Design review of the part shown in the three views and the two pictorial views. Dimensions are in mm from the part's minimum x, y and z. A direction names the side the tool comes from. Coordinates: 2 decimals unless noted, no trailing zeros. Write each loop counter-clockwise with the first axis right and the second up, starting at its lowest first coordinate (ties: lowest second). Pieces come first, ordered by that corner, then holes. Notation, with made-up numbers: (21, 16.25) -> (57, 16.25) arc R13 ccw to (57, 39.25) -> close; hole circle Ø2 at (77.5, -8). An arc over 180 degrees is marked (long way). Answer in a Markdown table with one row per item. Add a question column.
Item 1: Take a section at C-C, the plane z = 9.75. Write out the cut boundary in (x, y).
Item 2: For the marked faces 5 and 6, list the 3-axis set-ups (+Z, -Z, +X, -X, +Y, -Y) from which the entire face can be reached by the end or side of a thin tool; tool diameter is ignored.
Item 3: Draft analysis for pull direction X (two halves, no side actions). For the marked faces 1, 2, 3 and 4, state which applies: released by +X, released by -X, zero draft, split by the parting line, or undercut.
Item 4: To check wall thickness, follow line 1 (X direction, y = 83, z = 13); line 2 (Y direction, x = 57.15, z = 1.55). State the ranges of each line that lie inside material, in increasing order.
Item 5: Take a section at A-A, the plane y = 57.15. Write out the cut boundary in (x, z).
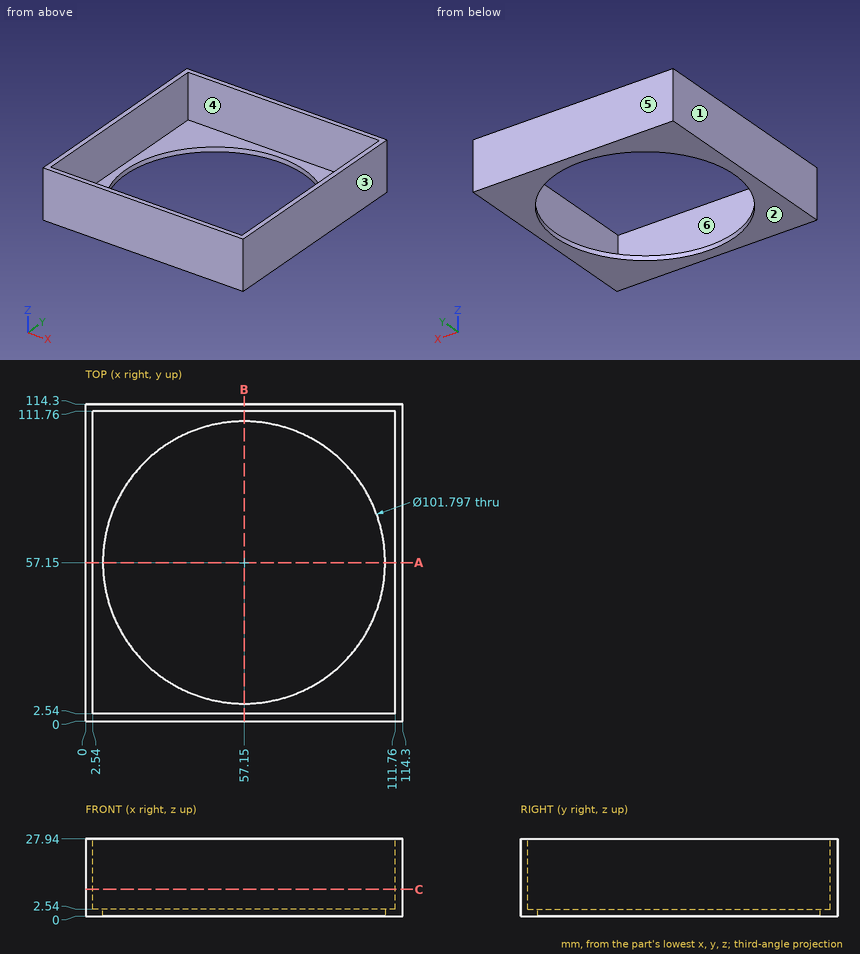
Answers:
| question | item | result |
|---|---|---|
| 1 | outline | (0, 0) -> (114.3, 0) -> (114.3, 114.3) -> (0, 114.3) -> close; hole (2.54, 2.54) -> (111.76, 2.54) -> (111.76, 111.76) -> (2.54, 111.76) -> close |
| 2 | face 5 | +Z, -Z, +X, -X, +Y |
| 2 | face 6 | +Z |
| 3 | face 1 | released by -X |
| 3 | face 2 | zero draft |
| 3 | face 3 | released by +X |
| 3 | face 4 | undercut |
| 4 | line 1 | x = 0 to 2.54, 111.76 to 114.3 |
| 4 | line 2 | y = 0 to 6.25, 108.05 to 114.3 |
| 5 | outline | (0, 0) -> (6.25, 0) -> (6.25, 2.54) -> (2.54, 2.54) -> (2.54, 27.94) -> (0, 27.94) -> close; (108.05, 0) -> (114.3, 0) -> (114.3, 27.94) -> (111.76, 27.94) -> (111.76, 2.54) -> (108.05, 2.54) -> close |
